from build123d import *

# Parameters (mm, degrees)
SKETCH1_W           = 42
SKETCH1_H           = 42
BOSS_EXTRUDE1_DEPTH = 2.54
SKETCH2_W           = 42
SKETCH2_H           = 42
BOSS_EXTRUDE2_DEPTH = 9
SKETCH13_R          = 3.25
BOSS_EXTRUDE6_DEPTH = 13
SKETCH9_R           = 6.25
SKETCH9_R_2         = 2.05
BOSS_EXTRUDE5_DEPTH = 6.5
SKETCH10_R          = 2.05
CUT_EXTRUDE1_DEPTH  = 8
SKETCH12_W          = 17.78
SKETCH12_H          = 2
CUT_EXTRUDE2_DEPTH  = 4
FILLET1_R           = 3
FILLET2_R           = 0.5
FILLET3_R           = 3


with BuildPart() as part:
    # Sketch1 → Boss-Extrude1 (new body)
    with BuildSketch(Plane(origin=(0, 0, 0), x_dir=(1, 0, 0), z_dir=(0, 1, 0))):
        Rectangle(SKETCH1_W, SKETCH1_H)
    extrude(amount=BOSS_EXTRUDE1_DEPTH)

    # Sketch2 → Boss-Extrude2 (add)
    with BuildSketch(Plane(origin=(0, 2.54, 0), x_dir=(1, 0, 0), z_dir=(0, 1, 0))):
        Rectangle(SKETCH2_W, SKETCH2_H)
        with BuildLine():
            Line((-17, 11.522774425), (-17, -11.522774425))
            ThreePointArc((-17, -11.522774425), (-16.869274473, -11.859874356), (-16.545454545, -12.020704023))
            ThreePointArc((-16.545454545, -12.020704023), (-13.464466094, -13.464466094), (-12.020704023, -16.545454545))
            ThreePointArc((-12.020704023, -16.545454545), (-11.859874356, -16.869274473), (-11.522774425, -17))
            Line((-11.522774425, -17), (11.522774425, -17))
            ThreePointArc((11.522774425, -17), (11.859874356, -16.869274473), (12.020704023, -16.545454545))
            ThreePointArc((12.020704023, -16.545454545), (13.464466094, -13.464466094), (16.545454545, -12.020704023))
            ThreePointArc((16.545454545, -12.020704023), (16.869274473, -11.859874356), (17, -11.522774425))
            Line((17, -11.522774425), (17, 11.522774425))
            ThreePointArc((17, 11.522774425), (16.869274473, 11.859874356), (16.545454545, 12.020704023))
            ThreePointArc((16.545454545, 12.020704023), (13.464466094, 13.464466094), (12.020704023, 16.545454545))
            ThreePointArc((12.020704023, 16.545454545), (11.859874356, 16.869274473), (11.522774425, 17))
            Line((11.522774425, 17), (-11.522774425, 17))
            ThreePointArc((-11.522774425, 17), (-11.859874356, 16.869274473), (-12.020704023, 16.545454545))
            ThreePointArc((-12.020704023, 16.545454545), (-13.464466094, 13.464466094), (-16.545454545, 12.020704023))
            ThreePointArc((-16.545454545, 12.020704023), (-16.869274473, 11.859874356), (-17, 11.522774425))
        make_face(mode=Mode.SUBTRACT)
    extrude(amount=BOSS_EXTRUDE2_DEPTH)

    # Sketch13 → Boss-Extrude6 (add, symmetric)
    with BuildSketch(Plane(origin=(0, 0, 0), x_dir=(0, 0, -1), z_dir=(1, 0, 0))):
        with BuildLine():
            Line((-7.5, 0), (-5.927131841, -10))
            ThreePointArc((-5.927131841, -10), (0, -15.067740305), (5.927131841, -10))
            Line((5.927131841, -10), (7.5, 0))
            Line((7.5, 0), (-7.5, 0))
        make_face()
        with Locations((0, -9.067740305)):
            Circle(SKETCH13_R, mode=Mode.SUBTRACT)
    extrude(amount=BOSS_EXTRUDE6_DEPTH, both=True)

    # Sketch9 → Boss-Extrude5 (add)
    with BuildSketch(Plane(origin=(0, 2.54, 0), x_dir=(1, 0, 0), z_dir=(0, 1, 0))):
        with Locations((8, 0)):
            Circle(SKETCH9_R)
        with Locations((8, 0)):
            Circle(SKETCH9_R_2, mode=Mode.SUBTRACT)
        with Locations((-8, 0)):
            Circle(SKETCH9_R)
        with Locations((-8, 0)):
            Circle(SKETCH9_R_2, mode=Mode.SUBTRACT)
    extrude(amount=BOSS_EXTRUDE5_DEPTH)

    # Sketch10 → Cut-Extrude1 (cut)
    with BuildSketch(Plane(origin=(0, 11.54, 0), x_dir=(1, 0, 0), z_dir=(0, 1, 0))):
        with Locations((-17, 17)):
            Circle(SKETCH10_R)
        with Locations((17, 17)):
            Circle(SKETCH10_R)
        with Locations((-17, -17)):
            Circle(SKETCH10_R)
        with Locations((17, -17)):
            Circle(SKETCH10_R)
    extrude(amount=-CUT_EXTRUDE1_DEPTH, mode=Mode.SUBTRACT)

    # Sketch12 → Cut-Extrude2 (cut)
    with BuildSketch(Plane(origin=(0, 0, -21), x_dir=(-1, 0, 0), z_dir=(0, 0, -1))):
        with Locations((0, 10.54)):
            Rectangle(SKETCH12_W, SKETCH12_H)
    extrude(amount=-CUT_EXTRUDE2_DEPTH, mode=Mode.SUBTRACT)

    # Fillet1
    fillet1_edges = [part.edges().sort_by_distance(p)[0] for p in [
        (21, 5.77, 21),
        (-21, 5.77, 21),
        (-21, 5.77, -21),
        (21, 5.77, -21),
    ]]
    fillet(fillet1_edges, radius=FILLET1_R)

    # Fillet2
    fillet2_edges = [part.edges().sort_by_distance(p)[0] for p in [
        (8.89, 10.54, -21),
        (0, 9.54, -21),
        (-8.89, 10.54, -21),
        (0, 9.54, -17),
        (-8.89, 9.54, -19),
        (-8.89, 10.54, -17),
        (8.89, 10.54, -17),
        (8.89, 9.54, -19),
    ]]
    fillet(fillet2_edges, radius=FILLET2_R)

    # Fillet3
    fillet3_edges = [part.edges().sort_by_distance(p)[0] for p in [
        (0, 0, -7.5),
        (0, 0, 7.5),
    ]]
    fillet(fillet3_edges, radius=FILLET3_R)


solid = part.part
Could you check a few things on this model? Use its own coordinates, in mm. A direction names the side the tool comes from. Coordinates: 2 decimals unless noted, no trailing zeros. Loops run counter-clockwise (first coordinate to the right, second up) from the corner with the lowest first, then second, coordinate; pieces in that order, holes last. Notation, with made-up numbers: (75.25, 15) -> (111.25, 15) arc R3 ccw to (111.25, 19) -> close; hole circle Ø4 at (59, -14.5). An arc over 180 degrees is marked (long way). Answer in a Markdown table with one row per item.
(1) Imagine slicing it at A-A (y = 4.5). Give the number of separate pieces and of enclosed holes in the cut face, plus the area to 3 significant figures.
Results found:
| item | result |
|---|---|
| separate pieces | 3 |
| enclosed holes | 7 |
| area | 845 mm^2 |
(2) Imagine slicing it at D-D (y = -11.5). List the corners of the cut face in (x, z) for me, plus the area to 3 significant figures.
Results found:
| item | result |
|---|---|
| outline | (-13, -5.48) -> (13, -5.48) -> (13, -2.16) -> (-13, -2.16) -> close; (-13, 2.16) -> (13, 2.16) -> (13, 5.48) -> (-13, 5.48) -> close |
| area | 173 mm^2 |
(3) For faces 1 (the face through (-5, 9.04, 0)), 2 (the face through (-13, -4, 0)), 3 (the face through (0, 0, -14)), which set-ups out of +Z, -Z, +X, -X, +Y, -Y let a thin tool reach every point of the face, with its end or its side?
Results found:
| item | result |
|---|---|
| face 1 | +Y |
| face 2 | +Z, -Z, -X, -Y |
| face 3 | -Y |
(4) If I drill on probe 1 along Z at (x, y) = (8, 7); probe 2 along X at (y, z) = (5.25, 0); probe 3 along Y at (x, z) = (1, 0), over which ranges is the centre line in solid material (lowest first)?
Results found:
| item | result |
|---|---|
| probe 1 | z = -21 to -17, -6.25 to -2.05, 2.05 to 6.25, 17 to 21 |
| probe 2 | x = -21 to -17, -14.25 to -10.05, -5.95 to -1.75, 1.75 to 5.95, 10.05 to 14.25, 17 to 21 |
| probe 3 | y = -15.07 to -12.32, -5.82 to 2.54 |
(5) Will these pins go through, and if not, where does the flat tip stop? pin 1 Ø2.5 at (x, z) = (-8, 0) entering from +Y; pin 2 Ø2 at (y, z) = (-7, -3.5) entering from +X; pin 3 Ø4.5 at (y, z) = (-9.5, 1.5) entering from -X.
Results found:
| item | result |
|---|---|
| pin 1 | stops at y = 2.54 |
| pin 2 | stops at x = 13 |
| pin 3 | stops at x = -13 |
(6) Imagine slicing it at C-C (x = -2.5). List the corners of the cut face in (y, z) for me.
Results found:
| item | result |
|---|---|
| outline | (-10, -5.93) -> (-2.53, -7.1) arc R3 cw to (0, -10.07) -> (0, -21) -> (9.04, -21) arc R0.5 ccw to (9.54, -20.5) -> (9.54, -17.5) arc R0.5 ccw to (9.04, -17) -> (2.54, -17) -> (2.54, -2.97) -> (9.04, -2.97) -> (9.04, 2.97) -> (2.54, 2.97) -> (2.54, 17) -> (11.54, 17) -> (11.54, 21) -> (0, 21) -> (0, 10.07) arc R3 cw to (-2.53, 7.1) -> (-10, 5.93) arc R6 ccw to start; hole circle Ø6.5 at (-9.07, 0) |
(7) Thinking about a two-plate mould opening in X: for faces 4 (the face through (0, 11.54, 18)), 5 (the face through (20.1, 5.69, -20.14)), 6 (the face through (13.5, 6.98, -13.43)), which applies, released by +X, released by -X, zero draft, split by the parting line, or undercut?
Results found:
| item | result |
|---|---|
| face 4 | zero draft |
| face 5 | released by +X |
| face 6 | undercut |
